Autodesk Inventor part; units mm, degrees
ref_plane "YZ Plane" through (0, 0, 0) normal (1, 0, 0) x (0, 1, 0)
ref_plane "XZ Plane" through (0, 0, 0) normal (0, 1, 0) x (-1, 0, 0)
ref_plane "XY Plane" through (0, 0, 0) normal (0, 0, 1) x (1, 0, 0)
sketch "Sketch1" plane through (0, 0, 0) normal (1, 0, 0) x (0, 1, 0)
  line L0 (0, 0) -> (79.6447, 0)
  line L1 (140, 60.3553) -> (140, 185)
  line L2 (115, 210) -> (50, 210)
  line L3 (0, 110) -> (0, 0)
  arc A0 (140, 185) -> (115, 210) centre (115, 185) ccw
  line L4 (50, 210) -> (50, 110)
  line L5 (0, 110) -> (50, 110)
  circle A1 centre (115, 185) radius 5
  circle A2 centre (115, 150) radius 5
  circle A3 centre (60, 122) radius 5
  circle A4 centre (50, 95) radius 5
  line L6 (132.6777, 42.6777) -> (97.3223, 7.3223)
  arc A5 (132.6777, 42.6777) -> (140, 60.3553) centre (115, 60.3553) ccw
  arc A6 (79.6447, 0) -> (97.3223, 7.3223) centre (79.6447, 25) ccw
  circle A7 centre (15, 82.5) radius 5
  circle A8 centre (15, 27.5) radius 5
  point P0 (140, 210)
  point P1 (90, 0)
  dimension "d2" = 25
  dimension "d3" = 90
  dimension "d4" = 110
  dimension "d5" = 140
  dimension "d6" = 10
  dimension "d7" = 88
  dimension "d8" = 10
  dimension "d9" = 15
  dimension "d10" = 25
  dimension "d11" = 35
  dimension "d12" = 25
  dimension "d13" = 50
  dimension "d14" = 45
  dimension "d15" = 210
  dimension "d16" = 25
  dimension "d17" = 25
  dimension "d20" = 55
  dimension "d21" = 27.5
  dimension "d22" = 35
  dimension "d23" = 10
extrude "Extrusion1" add sketch "Sketch1" along normal blind 15.875
properties part number "bodytoppart" material "Steel, Mild"
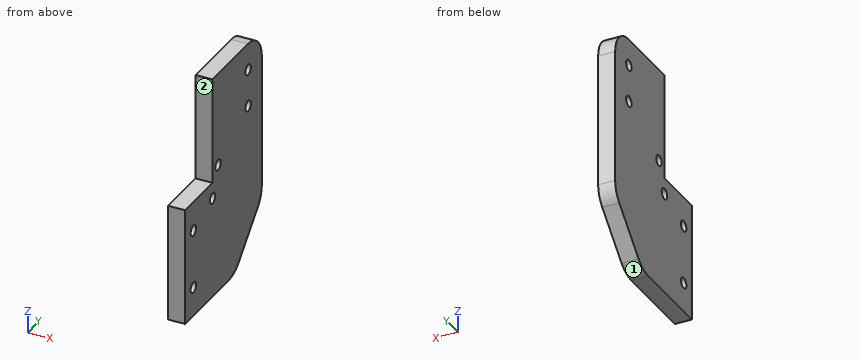
The model under review builds one solid part; all positions refer to its coordinate system, in mm. Face numbers are marked on the shaded views. A direction names the side the tool comes from. Coordinates: 2 decimals unless noted, no trailing zeros. Loops run counter-clockwise (first coordinate to the right, second up) from the corner with the lowest first, then second, coordinate; pieces in that order, holes last. Notation, with made-up numbers: (80, 84) -> (106, 84) arc R24 cw to (106, 122) -> close; hole circle Ø6 at (71, 8). An arc over 180 degrees is marked (long way). Use a Markdown table: item, result. Add a question column.
1. Clearance check with flat-ended pins moving along their axes: pin 1 Ø12 at (y, z) = (15, 72) entering from -X; pin 2 Ø8 at (y, z) = (15, 82.5) entering from -X; pin 3 Ø8 at (x, z) = (12, 152.5) entering from -Y. State where each tip first meets the part, or that it passes through.
2. Add section D-D on y = 60. Write out the cut boundary in (x, z) (3 decimals), plus the area to 4 significant figures.
3. Add section B-B on y = 15. Write out the cut boundary in (x, z) (3 decimals).
4. To check wall thickness, follow line 1 (Z direction, x = 6, y = 15); line 2 (Z direction, x = 10.5, y = 115); line 3 (Z direction, x = 7.5, y = 60). State the ranges of each line that lie inside material, in increasing order.
5. Machinability: for the marked faces 1 and 2, which of the approach directions +Z, -Z, +X, -X, +Y, -Y give a long, thin tool a straight path to every point of the face, cutting with its end or side? Answer none if there is none.
6. Add section C-C on x = 8. Write out the cut boundary in (y, z).
7. Add section A-A on z = 150. Write out the cut boundary in (x, y) (3 decimals).
Returned:
| question | item | result |
|---|---|---|
| 1 | pin 1 | stops at x = 0 |
| 1 | pin 2 | passes through |
| 1 | pin 3 | stops at y = 50 |
| 2 | outline | (0, 0) -> (15.875, 0) -> (15.875, 117) -> (0, 117) -> close; (0, 127) -> (15.875, 127) -> (15.875, 210) -> (0, 210) -> close |
| 2 | area | 3,175 mm² |
| 3 | outline | (0, 0) -> (15.875, 0) -> (15.875, 22.5) -> (0, 22.5) -> close; (0, 32.5) -> (15.875, 32.5) -> (15.875, 77.5) -> (0, 77.5) -> close; (0, 87.5) -> (15.875, 87.5) -> (15.875, 110) -> (0, 110) -> close |
| 4 | line 1 | z = 0 to 22.5, 32.5 to 77.5, 87.5 to 110 |
| 4 | line 2 | z = 25 to 145, 155 to 180, 190 to 210 |
| 4 | line 3 | z = 0 to 117, 127 to 210 |
| 5 | face 1 | -Z, +X, -X, +Y |
| 5 | face 2 | +Z, +X, -X, -Y |
| 6 | outline | (0, 0) -> (79.64, 0) arc R25 ccw to (97.32, 7.32) -> (132.68, 42.68) arc R25 ccw to (140, 60.36) -> (140, 185) arc R25 ccw to (115, 210) -> (50, 210) -> (50, 110) -> (0, 110) -> close; hole circle Ø10 at (15, 27.5); hole circle Ø10 at (15, 82.5); hole circle Ø10 at (50, 95); hole circle Ø10 at (60, 122); hole circle Ø10 at (115, 150); hole circle Ø10 at (115, 185) |
| 7 | outline | (0, 50) -> (15.875, 50) -> (15.875, 110) -> (0, 110) -> close; (0, 120) -> (15.875, 120) -> (15.875, 140) -> (0, 140) -> close |
